Build history of the part. All positions in model axes, mm. A direction names the side the tool comes from. Coordinates: 2 decimals unless noted, no trailing zeros. Order: outer loops, then holes, each group sorted by start corner. A loop starts at its lowest first (then second) coordinate and runs counter-clockwise, first axis right, second up. Notation, with made-up numbers: (62.5, 21.25) -> (113.5, 21.25) arc R18 cw to (113.5, 28.25) -> close; hole circle Ø11 at (47.5, -36). An arc over 180 degrees is marked (long way). Write each question's results on one line, items separated by ' | '.
from build123d import *

# Parameters (mm, degrees)
F1_DEPTH = 6


with BuildPart() as f1:
    # F0 (on Front) → F1 (new body)
    with BuildSketch(Plane.XZ):
        with BuildLine():
            Line((-19.5, 0), (-5, 0))
            ThreePointArc((-5, 0), (-1.464466, 1.464466), (0, 5))
            Line((0, 5), (0, 75))
            ThreePointArc((0, 75), (-1.464466, 78.535534), (-5, 80))
            Line((-5, 80), (-75, 80))
            ThreePointArc((-75, 80), (-78.535534, 78.535534), (-80, 75))
            Line((-80, 75), (-80, 5))
            ThreePointArc((-80, 5), (-78.535534, 1.464466), (-75, 0))
            Line((-75, 0), (-54.5, 0))
            Line((-54.5, 0), (-54.5, 5))
            Line((-54.5, 5), (-70, 5))
            ThreePointArc((-70, 5), (-73.535534, 6.464466), (-75, 10))
            Line((-75, 10), (-75, 70))
            ThreePointArc((-75, 70), (-73.535534, 73.535534), (-70, 75))
            Line((-70, 75), (-10, 75))
            ThreePointArc((-10, 75), (-6.464466, 73.535534), (-5, 70))
            Line((-5, 70), (-5, 10))
            ThreePointArc((-5, 10), (-6.464466, 6.464466), (-10, 5))
            Line((-10, 5), (-19.5, 5))
            Line((-19.5, 5), (-19.5, 0))
        make_face()
    extrude(amount=F1_DEPTH)


solid = f1.part
Item 1: Tool access for faces 4 (the flat face through (-19.5, -3, 3)), 5 (the flat face through (-62, -3, 5)), 6 (the cylindrical face through (-78, -3, 79)): list every direction of +Z, -Z, +X, -X, +Y, -Y with a clear straight run to the whole face (end or side of a thin tool).
Answer:
face 4: -Z, +Y, -Y | face 5: +Y, -Y | face 6: +Z, -X, +Y, -Y
Item 2: Slice it at C-C, the plane y = -1.3. List the corners of the cut face in (x, z).
Answer:
outline: (-80, 5) arc R5 ccw to (-75, 0) -> (-54.5, 0) -> (-54.5, 5) -> (-70, 5) arc R5 cw to (-75, 10) -> (-75, 70) arc R5 cw to (-70, 75) -> (-10, 75) arc R5 cw to (-5, 70) -> (-5, 10) arc R5 cw to (-10, 5) -> (-19.5, 5) -> (-19.5, 0) -> (-5, 0) arc R5 ccw to (0, 5) -> (0, 75) arc R5 ccw to (-5, 80) -> (-75, 80) arc R5 ccw to (-80, 75) -> close
Item 3: Drill centre lines: line 1 (X direction, y = -3.9, z = 35); line 2 (Z direction, x = -14.5, y = -5.1); line 3 (Z direction, x = -34.5, y = -4.8). Where is each one in solid material? Low to high. Write a range as from..to.
Answer:
line 1: x = -80..-75, -5..0 | line 2: z = 0..5, 75..80 | line 3: z = 75..80
Item 4: Slice it at B-B, the plane z = 60. List the corners of the cut face in (x, y), and give its area (3 significant figures).
Answer:
outline: (-80, -6) -> (-75, -6) -> (-75, 0) -> (-80, 0) -> close; (-5, -6) -> (0, -6) -> (0, 0) -> (-5, 0) -> close | area: 60.0 mm^2
Item 5: Pull direction X, two halves, no side cores. Call faces 1 (the cylindrical face through (-74, -3, 73)), 2 (the flat face through (-80, -3, 40)), 3 (the cylindrical face through (-1, -3, 78)): released by +X, released by -X, zero draft, split by the parting line, or undercut.
Answer:
face 1: undercut | face 2: released by -X | face 3: released by +X
Item 6: Pin check, flat tips, straight feed: pin 1 (2.5 mm diameter, centred on y = -2, z = 2, fed in from -X); pin 2 (8 mm diameter, centred on x = -11, z = 30.5, fed in from +Y). Stop position of each tip, or through.
Answer:
pin 1: stops at x = -79.68 | pin 2: passes through
Item 7: Slice it at D-D, the plane x = -32.5. List the corners of the cut face in (y, z), and give its area (3 significant figures).
Answer:
outline: (-6, 75) -> (0, 75) -> (0, 80) -> (-6, 80) -> close | area: 30.0 mm^2
Item 8: Slice it at A-A, the plane x = -63.5. List the corners of the cut face in (y, z).
Answer:
outline: (-6, 0) -> (0, 0) -> (0, 5) -> (-6, 5) -> close; (-6, 75) -> (0, 75) -> (0, 80) -> (-6, 80) -> close
